Build history of the part. All positions in model axes, mm. A direction names the side the tool comes from. Give positions to 0.01 mm unless a question says otherwise; leave off trailing zeros. Order: outer loops, then holes, each group sorted by start corner. A loop starts at its lowest first (then second) coordinate and runs counter-clockwise, first axis right, second up. Notation, with made-up numbers: (49, 13.25) - (83, 13.25) arc R17 cw to (83, 44.25) - close; hole circle Ø1 at (42.25, 27.5). An arc over 180 degrees is marked (long way). Use a Markdown table: item, result. Add a question column.
(1) Which spindle directions (+Z, -Z, +X, -X, +Y, -Y) get a long thin tool onto all of the face, cutting with end or side? Do faces 1 (the face through (8.5, -1, 0.5)), 2 (the face through (5, -3, 1)), 3 (the face through (1, -4.5, 0.5)). Say none if no direction does.
(2) Slice it at C-C (z = 0.85). Write the cut outline in (x, y).
(3) Mould opens along X. For faces 4 (the face through (0.285, -7.199, 0.493)), 5 (the face through (5.4, -7.5, 0.5)), 6 (the face through (10.699, -7.215, 0.493)), 7 (the face through (10, -4.5, 0.5)) say: +X half, -X half, draft (parallel to the pull), parting line (faces both ways), or undercut.
(4) Slice it at B-B (x = 6.5). Write the cut outline in (y, z).
(5) Slice it at A-A (y = -4.5). Write the cut outline in (x, z).
(6) Flat gauge pin, fed straight in: pin 1 (1.5 mm diameter, centred on x = 6.5, y = -4.5, fed in from -Z). Where does the tip first touch, or does it go through?
(7) Slice it at D-D (z = 0.2). Write the cut outline in (x, y).
(8) Wall check: line 1 (X direction, y = -4.5, z = 0.15); line 2 (Y direction, x = 2, z = 0.6); line 3 (Y direction, x = 8.25, z = 0.7). Give the ranges that are in metal, low to high.
from build123d import *

# Parameters (mm, degrees)
EXTRUDE074_DEPTH = 1
EXTRUDE075_DEPTH = 15
EXTRUDE073_DEPTH = 1


with BuildPart() as extrude074:
    # Sketch271 → Extrude074 (new body)
    with BuildSketch(Plane.XY):
        with BuildLine():
            Line((2, -5.5), (9, -5.5))
            ThreePointArc((9, -5.5), (10, -4.5), (9, -3.5))
            Line((2, -3.5), (9, -3.5))
            ThreePointArc((2, -3.5), (1, -4.5), (2, -5.5))
        make_face()
    extrude(amount=EXTRUDE074_DEPTH)


with BuildPart() as extrude075:
    # Sketch272 → Extrude075 (new body)
    with BuildSketch(Plane.YZ):
        with BuildLine():
            ThreePointArc((-0.5, 0), (-0.146447, 0.146447), (0, 0.5))
            Line((0, 0.5), (0, 0))
            Line((-0.5, 0), (0, 0))
        make_face()
    extrude(amount=EXTRUDE075_DEPTH)


with BuildPart() as cut045:
    # Sketch270 → Extrude073 (new body)
    with BuildSketch(Plane(origin=(0, -0.5, 0), x_dir=(1, 0, 0), z_dir=(0, 0, 1))):
        with BuildLine():
            ThreePointArc((0, -6), (0.292893, -6.707107), (1, -7))
            Line((1, -7), (10, -7))
            ThreePointArc((10, -7), (10.707107, -6.707106), (11, -6))
            Line((11, -6), (11, -1.5))
            ThreePointArc((11, -1.5), (10.707107, -0.792893), (10, -0.5))
            Line((10, -0.5), (7, -0.5))
            Line((7, -0.5), (7, 0.5))
            Line((7, 0.5), (0, 0.5))
            Line((0, 0.5), (0, -6))
        make_face()
    extrude(amount=EXTRUDE073_DEPTH)

    # Cut044: cut Extrude075
    add(extrude075.part, mode=Mode.SUBTRACT)

    # Cut045: cut Extrude074
    add(extrude074.part, mode=Mode.SUBTRACT)


solid = cut045.part
Solution:
| question | item | result |
|---|---|---|
| 1 | face 1 | +Z, -Z, +X, +Y |
| 1 | face 2 | +Z, +X, -X, +Y, -Y |
| 1 | face 3 | +Z, -Z |
| 2 | outline | (0, -6.5) arc R1 ccw to (1, -7.5) - (10, -7.5) arc R1 ccw to (11, -6.5) - (11, -2) arc R1 ccw to (10, -1) - (7, -1) - (7, 0) - (0, 0) - close; hole (2, -5.5) - (9, -5.5) arc R1 ccw to (9, -3.5) - (2, -3.5) arc R1 ccw to start |
| 3 | face 4 | -X half |
| 3 | face 5 | draft |
| 3 | face 6 | +X half |
| 3 | face 7 | undercut |
| 4 | outline | (-7.5, 0) - (-5.5, 0) - (-5.5, 1) - (-7.5, 1) - close; (-3.5, 0) - (-0.5, 0) arc R0.5 ccw to (0, 0.5) - (0, 1) - (-3.5, 1) - close |
| 5 | outline | (0, 0) - (1, 0) - (1, 1) - (0, 1) - close; (10, 0) - (11, 0) - (11, 1) - (10, 1) - close |
| 6 | pin 1 | through |
| 7 | outline | (0, -6.5) arc R1 ccw to (1, -7.5) - (10, -7.5) arc R1 ccw to (11, -6.5) - (11, -2) arc R1 ccw to (10, -1) - (7, -1) - (7, -0.1) - (0, -0.1) - close; hole (2, -5.5) - (9, -5.5) arc R1 ccw to (9, -3.5) - (2, -3.5) arc R1 ccw to start |
| 8 | line 1 | 0 to 1, 10 to 11 |
| 8 | line 2 | -7.5 to -5.5, -3.5 to 0 |
| 8 | line 3 | -7.5 to -5.5, -3.5 to -1 |
